Could you check a few things on this model? Use its own coordinates, in mm. Face numbers are marked on the shaded views. Round coordinates to 2 decimals unless told otherwise and drop trailing zeros. Write each question's results on one line, items separated by ' | '. Start each with the question number.
1. I'm going to push flat-ended pins straight in: pin 1 (8 mm diameter, centred on y = 10.5, z = 20.5, fed in from -X); pin 2 (2 mm diameter, centred on x = 7.17, y = -1.83, fed in from -Z); pin 3 (3 mm diameter, centred on y = -7.5, z = 22, fed in from -X); pin 4 (12 mm diameter, centred on x = -8, z = 16.5, fed in from -Y). Where does each tip first touch, or does it pass through?
2. Suppose I cut it at A-A on z = 16. Give the number of separate pieces and of enclosed holes in the cut face, and give its area (3 significant figures).
3. Please list where these lines run through material, in increasing order: L1, parallel to X at y = 1, z = 21.75; L2, parallel to Y at x = -1, z = 5; L3, parallel to X at y = -3.5, z = 16.25.
4. We'd pull the mould along Y, two halves only. Please class the marked faces 1, 2 and 3: released by +Y, released by -Y, zero draft, split by the parting line, or undercut.
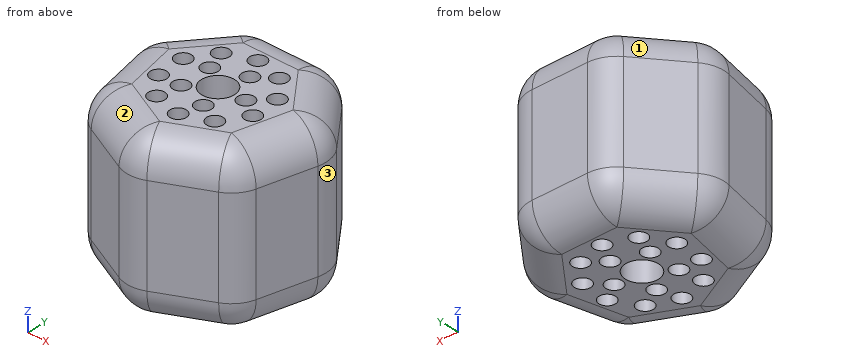
from build123d import *

# Parameters (mm, degrees)
F1_DEPTH = 25.4
F2_R     = 5.08
F3_R     = 5.08
F4_R     = 1.27
F4_R_2   = 2.54
F5_DEPTH = 37.084


with BuildPart() as f1:
    # F0 (on Top) → F1 (new body)
    with BuildSketch(Plane.XY):
        Polygon((6.806168, 14.133153), (-6.806168, 14.133153), (-15.29332, 3.4906), (-12.26429, -9.780445), (0, -15.686616), (12.26429, -9.780445), (15.29332, 3.4906), align=None)
    extrude(amount=F1_DEPTH)

    # F2
    f2_edges = [f1.edges().sort_by_distance(p)[0] for p in [
        (-12.26429, -9.780445, 12.7),
        (-15.29332, 3.4906, 12.7),
        (-6.806168, 14.133153, 12.7),
        (6.806168, 14.133153, 12.7),
        (15.29332, 3.4906, 12.7),
        (12.26429, -9.780445, 12.7),
        (0, -15.686616, 12.7),
    ]]
    fillet(f2_edges, radius=F2_R)

    # F3
    f3_edges = [f1.edges().sort_by_distance(p)[0] for p in [
        (0, 14.133153, 0),
        (0, 14.133153, 25.4),
        (6.563898, 13.630074, 25.4),
        (-6.563898, 13.630074, 25.4),
        (11.049744, 8.811876, 25.4),
        (-11.049744, 8.811876, 25.4),
        (14.748945, 3.36635, 25.4),
        (-14.748945, 3.36635, 25.4),
        (13.778805, -3.144922, 25.4),
        (-13.778805, -3.144922, 25.4),
        (11.827735, -9.432304, 25.4),
        (-11.827735, -9.432304, 25.4),
        (6.132145, -12.73353, 25.4),
        (-6.132145, -12.73353, 25.4),
        (0, -15.128241, 25.4),
    ]]
    fillet(f3_edges, radius=F3_R)

    # F4 (on face) → F5 (cut)
    with BuildSketch(Plane.XY.offset(25.4)):
        with Locations((0.477998, -7.379863)):
            Circle(F4_R)
        with Locations((-3.438198, -2.615431)):
            Circle(F4_R)
        with Locations((4.724483, -5.689474)):
            Circle(F4_R)
        with Locations((7.166376, -1.8259)):
            Circle(F4_R)
        with Locations((4.318873, 0.095006)):
            Circle(F4_R)
        with Locations((6.870957, 2.735106)):
            Circle(F4_R)
        with Locations((3.951066, 6.251395)):
            Circle(F4_R)
        with Locations((1.244249, 4.136851)):
            Circle(F4_R)
        Circle(F4_R_2)
        with Locations((1.424961, -4.078133)):
            Circle(F4_R)
        with Locations((-3.951066, -6.251395)):
            Circle(F4_R)
        with Locations((-6.870957, -2.735106)):
            Circle(F4_R)
        with Locations((-7.166376, 1.8259)):
            Circle(F4_R)
        with Locations((-3.549885, 2.461708)):
            Circle(F4_R)
        with Locations((-4.724483, 5.689474)):
            Circle(F4_R)
        with Locations((-0.477998, 7.379863)):
            Circle(F4_R)
    extrude(amount=-F5_DEPTH, mode=Mode.SUBTRACT)


solid = f1.part
Filled sheet:
1) pin 1: stops at x = -12.89 | pin 2: passes through | pin 3: stops at x = -13 | pin 4: stops at y = -14.72
2) separate pieces: 1 | enclosed holes: 16 | area: 571 mm^2
3) L1: x = -14.51 to -8.13, -6.2 to -2.33, 2.33 to 3.43, 5.21 to 14.51 | L2: y = -15.03 to -2.33, 2.33 to 6.22, 8.54 to 14.13 | L3: x = -13.7 to -7.88, -5.86 to -4.35, -2.53 to 0.29, 2.56 to 13.7
4) face 1: released by +Y | face 2: released by -Y | face 3: split by the parting line
